CAD build for the part. Positions are in the model's coordinates, mm. Coordinates: 2 decimals unless noted, no trailing zeros. Loops run counter-clockwise (first coordinate to the right, second up) from the corner with the lowest first, then second, coordinate; pieces in that order, holes last. Notation, with made-up numbers: (5.25, 16.5) -> (52.25, 16.5) arc R18 ccw to (52.25, 24.5) -> close; hole circle Ø6 at (65.25, -26). An arc over 180 degrees is marked (long way). Answer as CSV lines item,"result". Start each with the question number.
from build123d import *

# Parameters (mm, degrees)
CROQUIS1_W              = 50
CROQUIS1_H              = 50
SALIENTE_EXTRUIR1_DEPTH = 50
REDONDEO1_R             = 10


with BuildPart() as part:
    # Croquis1 → Saliente-Extruir1 (new body)
    with BuildSketch(Plane(origin=(0, 0, 0), x_dir=(0, 0, -1), z_dir=(1, 0, 0))):
        with Locations((25, 25)):
            Rectangle(CROQUIS1_W, CROQUIS1_H)
    extrude(amount=SALIENTE_EXTRUIR1_DEPTH)

    # Redondeo1
    redondeo1_edges = [part.edges().sort_by_distance(p)[0] for p in [
        (50, 50, -25),
        (0, 50, -25),
        (0, 0, -25),
        (50, 0, -25),
    ]]
    fillet(redondeo1_edges, radius=REDONDEO1_R)


solid = part.part
Item 1: Wall check: probe 1 along X at (y, z) = (6, -37); probe 2 along Y at (x, z) = (41, -23); probe 3 along X at (y, z) = (41.5, -33.5). Give the ranges that are in metal, low to high.
Item 2: Saw through at B-B (x = 5.5). Write the cut outline in (y, z).
Item 3: Saw through at A-A (z = -27). Write the cut outline in (x, y), plus the area to 3 significant figures.
Item 4: Flat gauge pin, fed straight in: pin 1 Ø10 at (x, y) = (20, 6.5) entering from +Z. Where does the tip first touch, or does it go through?
Item 5: Saw through at C-C (y = 43.5). Write the cut outline in (x, z).
Geometry check:
1,probe 1,"0.83 to 49.17"
1,probe 2,"0.05 to 49.95"
1,probe 3,"0.11 to 49.89"
2,outline,"(1.07, -50) -> (48.93, -50) -> (48.93, 0) -> (1.07, 0) -> close"
3,outline,"(0, 10) arc R10 ccw to (10, 0) -> (40, 0) arc R10 ccw to (50, 10) -> (50, 40) arc R10 ccw to (40, 50) -> (10, 50) arc R10 ccw to (0, 40) -> close"
3,area,"2,410 mm2"
4,pin 1,"z = 0"
5,outline,"(0.63, -50) -> (49.37, -50) -> (49.37, 0) -> (0.63, 0) -> close"
